```python
from build123d import *

# Parameters (mm, degrees)
SKETCH6_W            = 105
SKETCH6_H            = 83
BOSS_EXTRUDE3_DEPTH  = 4.5
SKETCH9_W            = 3
SKETCH9_H            = 101
CUT_EXTRUDE6_DEPTH   = 81
SKETCH10_W           = 1
SKETCH10_H           = 8
BOSS_EXTRUDE4_DEPTH  = 8
SKETCH11_W           = 1.226225524
SKETCH11_H           = 5
BOSS_EXTRUDE5_DEPTH  = 5
BOSS_EXTRUDE12_DEPTH = 1.226226
SKETCH27_W           = 15
SKETCH27_H           = 2
SKETCH27_W_2         = 41
SKETCH27_W_3         = 9
SKETCH27_H_2         = 15
BOSS_EXTRUDE20_DEPTH = 30
SKETCH28_W           = 1.5
SKETCH28_H           = 11
BOSS_EXTRUDE21_DEPTH = 3
SKETCH29_W           = 41
SKETCH29_H           = 2
BOSS_EXTRUDE22_DEPTH = 30
SKETCH30_W           = 2
SKETCH30_H           = 25
BOSS_EXTRUDE23_DEPTH = 50
SKETCH31_R           = 5
BOSS_EXTRUDE24_DEPTH = 35
DRAFT1_ANGLE         = -3.5
DRAFT3_ANGLE         = -3.5
SKETCH32_W           = 4
SKETCH32_H           = 15
BOSS_EXTRUDE25_DEPTH = 7
SKETCH33_W           = 4
SKETCH33_H           = 13
BOSS_EXTRUDE26_DEPTH = 3
SKETCH34_W           = 2
SKETCH34_H           = 3
BOSS_EXTRUDE27_DEPTH = 4
SKETCH35_W           = 2
SKETCH35_H           = 15
BOSS_EXTRUDE28_DEPTH = 3
SKETCH36_W           = 11.5
SKETCH36_H           = 2
BOSS_EXTRUDE29_DEPTH = 3


with BuildPart() as part:
    # Sketch6 → Boss-Extrude3 (new body)
    with BuildSketch(Plane(origin=(0, 0, 0), x_dir=(0, 0, -1), z_dir=(1, 0, 0))):
        with Locations((52.5, -41.5)):
            Rectangle(SKETCH6_W, SKETCH6_H)
    extrude(amount=BOSS_EXTRUDE3_DEPTH)

    # Sketch9 → Cut-Extrude6 (cut)
    with BuildSketch(Plane.XZ.offset(83)):
        with Locations((3, -52.5)):
            Rectangle(SKETCH9_W, SKETCH9_H)
    extrude(amount=-CUT_EXTRUDE6_DEPTH, mode=Mode.SUBTRACT)

    # Sketch10 → Boss-Extrude4 (add)
    with BuildSketch(Plane(origin=(0, 0, -2), x_dir=(-1, 0, 0), z_dir=(0, 0, -1))):
        with Locations((-4, -6)):
            Rectangle(SKETCH10_W, SKETCH10_H)
    extrude(amount=BOSS_EXTRUDE4_DEPTH)

    # Sketch11 → Boss-Extrude5 (add)
    with BuildSketch(Plane.XY.offset(-103)):
        with Locations((3.886887238, -4.5)):
            Rectangle(SKETCH11_W, SKETCH11_H)
    extrude(amount=BOSS_EXTRUDE5_DEPTH)

    # Sketch18 → Boss-Extrude12 (add)
    with BuildSketch(Plane(origin=(4.5, 0, 0), x_dir=(0, 0, -1), z_dir=(1, 0, 0))):
        Polygon((103, -12), (93, -2), (103, -2), align=None)
        Polygon((18, -2), (2, -2), (2, -18), align=None)
    extrude(amount=-BOSS_EXTRUDE12_DEPTH)

    # Sketch27 → Boss-Extrude20 (add)
    with BuildSketch(Plane.ZY):
        with Locations((-112.5, -54)):
            Rectangle(SKETCH27_W, SKETCH27_H)
        with Locations((-125.5, -19)):
            Rectangle(SKETCH27_W_2, SKETCH27_H)
        with Locations((-109.5, -1.5)):
            Rectangle(SKETCH27_W_3, SKETCH27_H_2)
        with Locations((-141.5, -1.5)):
            Rectangle(SKETCH27_W_3, SKETCH27_H_2)
    extrude(amount=-BOSS_EXTRUDE20_DEPTH)


with BuildPart() as boss_extrude20_piece_1:
    # of the separate pieces the step leaves, piece 1, a body of its own (boss_extrude20_pieces)
    add(part.part.solids().sort_by_distance((0, 0, 0))[0])



with BuildPart() as boss_extrude20_piece_2:
    # of the separate pieces the step leaves, piece 2, a body of its own (boss_extrude20_pieces)
    add(part.part.solids().sort_by_distance((0, 6, -146))[0])


with BuildPart() as boss_extrude20_piece_1_1:
    add(boss_extrude20_piece_1.part)

    add(boss_extrude20_piece_2.part)  # Boss-Extrude21 merges Boss-Extrude20 piece 2
    # Sketch28 → Boss-Extrude21 (add)
    with BuildSketch(Plane(origin=(30, 0, 0), x_dir=(0, 0, -1), z_dir=(1, 0, 0))):
        with Locations((145.25, -14.5)):
            Rectangle(SKETCH28_W, SKETCH28_H)
        with Locations((105.75, -14.5)):
            Rectangle(SKETCH28_W, SKETCH28_H)
    extrude(amount=-BOSS_EXTRUDE21_DEPTH)

    # Sketch29 → Boss-Extrude22 (add)
    with BuildSketch(Plane(origin=(30, 0, 0), x_dir=(0, 0, -1), z_dir=(1, 0, 0))):
        with Locations((125.5, 5)):
            Rectangle(SKETCH29_W, SKETCH29_H)
    extrude(amount=-BOSS_EXTRUDE22_DEPTH)

    # Sketch30 → Boss-Extrude23 (add)
    with BuildSketch(Plane(origin=(0, 0, -105), x_dir=(-1, 0, 0), z_dir=(0, 0, -1))):
        with Locations((-1, -45.5)):
            Rectangle(SKETCH30_W, SKETCH30_H)
    extrude(amount=BOSS_EXTRUDE23_DEPTH)

    # Sketch31 → Boss-Extrude24 (add)
    with BuildSketch(Plane(origin=(2, 0, 0), x_dir=(0, 0, -1), z_dir=(1, 0, 0))):
        with Locations(Location((149, -52, 0), (0, 0, 180))):
            Circle(SKETCH31_R)
        with Locations(Location((149, -39, 0), (0, 0, 180))):
            Circle(SKETCH31_R)
    extrude(amount=BOSS_EXTRUDE24_DEPTH)

    # Draft1
    draft1_faces = [boss_extrude20_piece_1_1.faces().sort_by_distance(p)[0] for p in [
        (19.5, -52, -154),
    ]]
    draft(draft1_faces, Plane(origin=(37, -52, -149), x_dir=(0, 0, 1), z_dir=(1, 0, 0)), DRAFT1_ANGLE)

    # Draft3
    draft3_faces = [boss_extrude20_piece_1_1.faces().sort_by_distance(p)[0] for p in [
        (19.5, -39, -154),
    ]]
    draft(draft3_faces, Plane(origin=(37, -39, -149), x_dir=(0, 0, 1), z_dir=(1, 0, 0)), DRAFT3_ANGLE)

    # Sketch32 → Boss-Extrude25 (add)
    with BuildSketch(Plane(origin=(2, 0, 0), x_dir=(0, 0, -1), z_dir=(1, 0, 0))):
        with Locations((149, -45.5)):
            Rectangle(SKETCH32_W, SKETCH32_H)
    extrude(amount=BOSS_EXTRUDE25_DEPTH)

    # Sketch33 → Boss-Extrude26 (add)
    with BuildSketch(Plane(origin=(37, 0, 0), x_dir=(0, 0, -1), z_dir=(1, 0, 0))):
        with Locations((149, -45.5)):
            Rectangle(SKETCH33_W, SKETCH33_H)
    extrude(amount=-BOSS_EXTRUDE26_DEPTH)

    # Sketch34 → Boss-Extrude27 (add)
    with BuildSketch(Plane(origin=(4.5, 0, 0), x_dir=(0, 0, -1), z_dir=(1, 0, 0))):
        with Locations((104, -81.5)):
            Rectangle(SKETCH34_W, SKETCH34_H)
    extrude(amount=BOSS_EXTRUDE27_DEPTH)

    # Sketch35 → Boss-Extrude28 (add)
    with BuildSketch(Plane(origin=(8.5, 0, 0), x_dir=(0, 0, -1), z_dir=(1, 0, 0))):
        with Locations((104, -87.5)):
            Rectangle(SKETCH35_W, SKETCH35_H)
    extrude(amount=BOSS_EXTRUDE28_DEPTH)

    # Sketch36 → Boss-Extrude29 (add)
    with BuildSketch(Plane(origin=(0, -95, 0), x_dir=(-1, 0, 0), z_dir=(0, -1, 0))):
        with Locations((-5.75, 104)):
            Rectangle(SKETCH36_W, SKETCH36_H)
    extrude(amount=BOSS_EXTRUDE29_DEPTH)


solid = boss_extrude20_piece_1_1.part
```
For this review, take the finished solid that the model builds, in its own axes (mm). A direction names the side the tool comes from. Coordinates: 2 decimals unless noted, no trailing zeros. Order: outer loops, then holes, each group sorted by start corner. A loop starts at its lowest first (then second) coordinate and runs counter-clockwise, first axis right, second up. Notation, with made-up numbers: (-12.5, -4) -> (16.5, -4) arc R19 cw to (16.5, 1) -> close; hole circle Ø11 at (0, 69.5). An arc over 180 degrees is marked (long way). Use CSV: the item, a comma, the result in double quotes. Start each with the question number.
Item 1: Insertion check: pin 1 (0.8 mm diameter, centred on y = -15.5, z = -145, fed in from -X); pin 2 (13 mm diameter, centred on x = 17, y = -3, fed in from +Z); pin 3 (2 mm diameter, centred on y = -10, z = -82, fed in from +X). Each pin has a flat end and moves straight along its axis. Give the tip position at first contact, or say it passes through.
Item 2: Draft analysis for pull direction Y (two halves, no side actions). For faces 4 (the face through (3, -2, -52)), 5 (the face through (3.274, -6, -99)), 6 (the face through (36, -46, -147)), state which applies: pulls with the +Y half, pulls with the -Y half, needs draft (parallel to the pull), parting line crosses it, or undercut.
Item 3: Wall thickness on probe 1 along Y at (x, z) = (18.5, -118); probe 2 along Y at (x, z) = (8, -108); probe 3 along Y at (x, z) = (17, -121): over which ranges is each line inside the solid? List them lowest first.
Item 4: For faces 1 (the face through (15, -4, -146)), 2 (the face through (5, -46, -151)), 3 (the face through (4, -10, -10)), list the 3-axis set-ups (+Z, -Z, +X, -X, +Y, -Y) from which the entire face can be reached by the end or side of a thin tool; tool diameter is ignored.
Item 5: We need section C-C, the plane y = -69. Give the boundary of the cut face in (x, z).
Item 6: We need section D-D, the plane z = -70.5. Give the boundary of the cut face in (x, y), then the cut area to 4 significant figures.
Item 7: We need section B-B, the plane x = 16.5. Give the boundary of the cut face in (y, z).
Item 8: We need section A-A, the plane z = -109. Give the boundary of the cut face in (x, y), then the cut area to 3 significant figures.
Derived:
1,pin 1,"stops at x = 27"
1,pin 2,"stops at z = -105"
1,pin 3,"stops at x = 1.5"
2,face 4,"pulls with the -Y half"
2,face 5,"needs draft"
2,face 6,"undercut"
3,probe 1,"y = -55 to -53, -20 to -18, 4 to 6"
3,probe 2,"y = -55 to -53, -20 to -18, -9 to 6"
3,probe 3,"y = -20 to -18, 4 to 6"
4,face 1,"-Z, +X, -X, +Y"
4,face 2,"-Z"
4,face 3,"+X, -Y"
5,outline,"(0, -105) -> (4.5, -105) -> (4.5, -103) -> (1.5, -103) -> (1.5, -2) -> (4.5, -2) -> (4.5, 0) -> (0, 0) -> close"
6,outline,"(0, -83) -> (1.5, -83) -> (1.5, -2) -> (4.5, -2) -> (4.5, 0) -> (0, 0) -> close"
6,area,"130.5 mm^2"
7,outline,"circle Ø7.49 at (-52, -149); (-55, -120) -> (-53, -120) -> (-53, -105) -> (-55, -105) -> close; circle Ø7.49 at (-39, -149); (-20, -146) -> (-18, -146) -> (-18, -105) -> (-20, -105) -> close; (-9, -146) -> (6, -146) -> (6, -105) -> (-9, -105) -> (-9, -114) -> (4, -114) -> (4, -137) -> (-9, -137) -> close"
8,outline,"(0, -58) -> (2, -58) -> (2, -55) -> (30, -55) -> (30, -53) -> (2, -53) -> (2, -33) -> (0, -33) -> close; (0, -20) -> (30, -20) -> (30, -18) -> (0, -18) -> close; (0, -9) -> (30, -9) -> (30, 6) -> (0, 6) -> close"
8,area,"616 mm^2"
